CAD build for the part. Positions are in the model's coordinates, mm. Give positions to 0.01 mm unless a question says otherwise; leave off trailing zeros. Loops run counter-clockwise (first coordinate to the right, second up) from the corner with the lowest first, then second, coordinate; pieces in that order, holes last. Notation, with made-up numbers: (-20, 35) -> (11, 35) arc R20 ccw to (11, 58) -> close; hole circle Ø8 at (48.25, 38). An arc over 180 degrees is marked (long way). Use one line per item in the form item = value.
```python
from build123d import *

# Parameters (mm, degrees)
SKETCH1_W                    = 736.6
SKETCH1_H                    = 101.6
BASE_FLANGE1_DEPTH           = 3.175
CUT_EXTRUDE2_DEPTH           = 3.175
EDGE_FLANGE1_STRIP_W         = 14.1732
EDGE_FLANGE1_STRIP_H         = 3.175
EDGE_FLANGE1_STRIP_CUT_DEPTH = 660.4
EDGE_FLANGE1_DEPTH           = 660.4
SKETCH12_R                   = 14.2875
SKETCH12_R_2                 = 4.7625
CUT_EXTRUDE3_DEPTH           = 373.35589998
SKETCH13_R                   = 3.175
CUT_EXTRUDE4_DEPTH           = 373.35589998


# Sheet-metal steps are written as plain solids
with BuildPart() as part:
    # Sketch1 → Base-Flange1 (new body)
    with BuildSketch(Plane.XY):
        Rectangle(SKETCH1_W, SKETCH1_H)
    extrude(amount=-BASE_FLANGE1_DEPTH)

    # Sketch11 → Cut-Extrude2 (cut)
    with BuildSketch(Plane.XY):
        Polygon((-368.3, -50.8), (-330.2, -50.8), (-368.3, -12.7), align=None)
        Polygon((368.3, -50.8), (330.2, -50.8), (368.3, -12.7), align=None)
    extrude(amount=-CUT_EXTRUDE2_DEPTH, mode=Mode.SUBTRACT)

    # Edge-Flange1 strip (across the edge) → Edge-Flange1 strip cut (cut)
    with BuildSketch(Plane(origin=(330.2, -50.8, -3.175), x_dir=(0, 1, 0), z_dir=(-1, 0, 0))):
        with Locations((-6.35, -1.5875)):
            Rectangle(EDGE_FLANGE1_STRIP_W, EDGE_FLANGE1_STRIP_H)
    extrude(amount=EDGE_FLANGE1_STRIP_CUT_DEPTH, mode=Mode.SUBTRACT)

    # Edge-Flange1 section (across the edge) → Edge-Flange1 (add)
    with BuildSketch(Plane(origin=(330.2, -50.8, -3.175), x_dir=(0, 1, 0), z_dir=(-1, 0, 0))):
        with BuildLine():
            Line((-3.175, 0.7366), (-3.175, 6.35))
            Line((-3.175, 6.35), (0, 6.35))
            Line((0, 6.35), (0, 0.7366))
            ThreePointArc((0, 0.7366), (0.215745145, 0.215745145), (0.7366, 0))
            Line((0.7366, 0), (0.7366, -3.175))
            ThreePointArc((0.7366, -3.175), (-2.029318885, -2.029318885), (-3.175, 0.7366))
        make_face()
    extrude(amount=EDGE_FLANGE1_DEPTH)

    # Sketch12 → Cut-Extrude3 (cut, through all)
    with BuildSketch(Plane.XY):
        with Locations((0, -24.6634)):
            Circle(SKETCH12_R)
        with Locations((-265.1125, -21.4884)):
            Circle(SKETCH12_R_2)
        with Locations((265.1125, -21.4884)):
            Circle(SKETCH12_R_2)
    extrude(amount=-CUT_EXTRUDE3_DEPTH, mode=Mode.SUBTRACT)

    # Sketch13 → Cut-Extrude4 (cut, through all)
    with BuildSketch(Plane.XY):
        with Locations((355.6, 38.1)):
            Circle(SKETCH13_R)
        with Locations((355.6, 12.7)):
            Circle(SKETCH13_R)
        with Locations((-355.6, 12.7)):
            Circle(SKETCH13_R)
        with Locations((-355.6, 38.1)):
            Circle(SKETCH13_R)
        with Locations((-213.36, 38.1)):
            Circle(SKETCH13_R)
        with Locations((-71.12, 38.1)):
            Circle(SKETCH13_R)
        with Locations((71.12, 38.1)):
            Circle(SKETCH13_R)
        with Locations((213.36, 38.1)):
            Circle(SKETCH13_R)
        with Locations((-132.584083533, -25.4)):
            Circle(SKETCH13_R)
        with Locations((132.584083533, -25.4)):
            Circle(SKETCH13_R)
    extrude(amount=-CUT_EXTRUDE4_DEPTH, mode=Mode.SUBTRACT)


solid = part.part
```
1. Drill centre lines: line 1 (Y direction, x = 355.6, z = -0.8) (3 decimals); line 2 (Z direction, x = 91.5, y = -45) (3 decimals); line 3 (Y direction, x = 36, z = -8) (3 decimals). Where is each one in solid material? Low to high.
Result sheet:
line_1 = -25.4 to 9.525, 15.875 to 34.925, 41.275 to 50.8
line_2 = -3.175 to 0
line_3 = -53.975 to -50.8
2. Mould opens along Y. For faces 1 (the cylindrical face through (-1.86, -10.497, -1.565)), 2 (the flat face through (-5, 1, -3.175)), 3 (the flat face through (349, -32, -2)) say: pulls with the +Y half, pulls with the -Y half, needs draft (parallel to the pull), parting line crosses it, or undercut.
Result sheet:
face_1 = undercut
face_2 = needs draft
face_3 = pulls with the -Y half
3. Cut at A-A, the plane x = 0. Write the cut outline in (y, z) (3 decimals), then the cut area to 3 significant figures.
Result sheet:
outline = (-53.975, -9.525) -> (-50.8, -9.525) -> (-50.8, -3.912) arc R0.737 cw to (-50.063, -3.175) -> (-38.951, -3.175) -> (-38.951, 0) -> (-50.063, 0) arc R3.912 ccw to (-53.975, -3.912) -> close; (-10.376, -3.175) -> (50.8, -3.175) -> (50.8, 0) -> (-10.376, 0) -> close
area = 259 mm^2
4. Cut at C-C, the plane z = -5.5. Write the cut outline in (x, y) (3 decimals), then the cut area to 3 significant figures.
Result sheet:
outline = (-330.2, -53.975) -> (330.2, -53.975) -> (330.2, -50.8) -> (-330.2, -50.8) -> close
area = 2,100 mm^2
5. Drop flat-ended pins along their axis: P1, Ø7.5, axis at x = -355.6, y = 38.1, coming from the +Z side; P2, Ø11, axis at x = 265.11, y = -21.49, coming from the -Z side (3 decimals); P3, Ø1, axis at y = -25.5, z = -2, coming from the +X side; P4, Ø4.5, axis at y = -52.5, z = -3, coming from the +X side. Give the stop position or say it passes through.
Result sheet:
P1 = 0
P2 = -3.175
P3 = 356
P4 = 330.75
6. Cut at B-B, the plane x = 297. Write the cut outline in (y, z) (3 decimals).
Result sheet:
outline = (-53.975, -9.525) -> (-50.8, -9.525) -> (-50.8, -3.912) arc R0.737 cw to (-50.063, -3.175) -> (50.8, -3.175) -> (50.8, 0) -> (-50.063, 0) arc R3.912 ccw to (-53.975, -3.912) -> close
